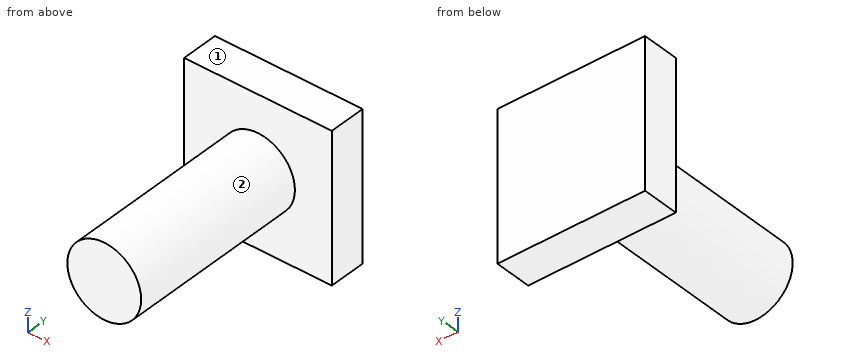
from build123d import *

# Parameters (mm, degrees)
SKETCH_1_W          = 20
SKETCH_1_H          = 20
EXTRUDE_1_DEPTH     = 30
SKETCH_3_W          = 20
SKETCH_3_H          = 20
SKETCH_3_R          = 5
CUT_EXTRUDE_1_DEPTH = 25


with BuildPart() as part:
    # Эскиз1 → Бобышка-Вытянуть1 (new body)
    with BuildSketch(Plane(origin=(0, 0, 0), x_dir=(1, 0, 0), z_dir=(0, 1, 0))):
        Rectangle(SKETCH_1_W, SKETCH_1_H)
    extrude(amount=EXTRUDE_1_DEPTH)

    # Эскиз3 → Вырез-Вытянуть1 (cut)
    with BuildSketch(Plane.XZ):
        Rectangle(SKETCH_3_W, SKETCH_3_H)
        Circle(SKETCH_3_R, mode=Mode.SUBTRACT)
    extrude(amount=-CUT_EXTRUDE_1_DEPTH, mode=Mode.SUBTRACT)


solid = part.part
Read the model definition and answer for the solid it produces. Units are mm, in the model's axes. Face numbers are marked on the shaded views. A direction names the side the tool comes from. Round coordinates to 2 decimals unless told otherwise and drop trailing zeros. Loops run counter-clockwise (first coordinate to the right, second up) from the corner with the lowest first, then second, coordinate; pieces in that order, holes last.
Q1. Each of these flat-tipped pins is pushed along its axis until it touches: pin 1 (10 mm diameter, centred on x = -5, y = 7.5, fed in from -Z); pin 2 (2 mm diameter, centred on y = 14.5, z = -6.5, fed in from -X); pin 3 (6 mm diameter, centred on x = 1, z = -2, fed in from -Y); pin 4 (4 mm diameter, centred on y = 15.5, z = -1.5, fed in from +X). Where does it stop, or does it pass through?
Q2. Section D-D on z = -8.5 is taken. Write down the section's boundary in (x, y).
Q3. Section A-A on x = 0 is taken. Write down the section's boundary in (y, z).
Q4. Section B-B on z = 3 is taken. Write down the section's boundary in (x, y), and give its area (3 significant figures).
Q5. Consider probe 1 along Y at (x, z) = (0.5, 9); probe 2 along Z at (x, y) = (3.25, 16); probe 3 along Z at (x, y) = (4.25, 6.75). Determine where each line is inside the solid, lowest interval first.
Q6. Section C-C on y = 17.25 is taken. Write down the section's boundary in (x, z).
Q7. Which of the six approach directions +Z, -Z, +X, -X, +Y, -Y give full straight-line access (tool end or side, diameter ignored) to the marked faces 1 and 2?
Output:
1. pin 1: stops at z = -5
1. pin 2: passes through
1. pin 3: stops at y = 0
1. pin 4: stops at x = 5
2. outline: (-10, 25) - (10, 25) - (10, 30) - (-10, 30) - close
3. outline: (0, -5) - (25, -5) - (25, -10) - (30, -10) - (30, 10) - (25, 10) - (25, 5) - (0, 5) - close
4. outline: (-10, 25) - (-4, 25) - (-4, 0) - (4, 0) - (4, 25) - (10, 25) - (10, 30) - (-10, 30) - close
4. area: 300 mm2
5. probe 1: y = 25 to 30
5. probe 2: z = -3.8 to 3.8
5. probe 3: z = -2.63 to 2.63
6. outline: circle Ø10 at (0, 0)
7. face 1: +Z, +X, -X, +Y, -Y
7. face 2: -Y
